Geometry check sheet. Reference: the model listing, model coordinates, mm. A direction names the side the tool comes from. Round coordinates to 2 decimals unless told otherwise and drop trailing zeros. Write each loop counter-clockwise with the first axis right and the second up, starting at its lowest first coordinate (ties: lowest second). Pieces come first, ordered by that corner, then holes. Notation, with made-up numbers: M 9.5,77 L 55.5,77 A27 cw 55.5,113 Z; hole C 79.5,6.25 d2. An arc over 180 degrees is marked long. Answer as CSV lines item,"result". Start each with the question number.
```python
from build123d import *

# Parameters (mm, degrees)
F1_DEPTH = 2
F3_DEPTH = 1


with BuildPart() as f1:
    # F0 (on Top) → F1 (new body)
    with BuildSketch(Plane.XY):
        Polygon((0, -11), (0, 0), (0, 11), (-2, 11), (-2, 2), (-8, 4.923089), (-8, 10.923089), (-12, 10.923089), (-12, 4.923089), (-29, 4.923089), (-46, 4.923089), (-46, 10.923089), (-50, 10.923089), (-50, 4.923089), (-60, 2), (-60, 10.923089), (-62, 10.923089), (-62, -10.923089), (-60, -10.923089), (-60, -2), (-50, -4.923089), (-50, -10.923089), (-46, -10.923089), (-46, -4.923089), (-29, -4.923089), (-12, -4.923089), (-12, -10.923089), (-8, -10.923089), (-8, -4.923089), (-2, -2), (-2, -11), align=None)
        Polygon((-60, 0), (-50, 2.923089), (-50, -2.923089), align=None, mode=Mode.SUBTRACT)
        Polygon((-12, 2.923089), (-12, 0), (-12, -2.923089), (-29, -2.923089), (-46, -2.923089), (-46, 0), (-46, 2.923089), (-29, 2.923089), align=None, mode=Mode.SUBTRACT)
        Polygon((-8, 2.923089), (-2, 0), (-8, -2.923089), (-8, 0), align=None, mode=Mode.SUBTRACT)
    extrude(amount=F1_DEPTH)

    # F2 (on face) → F3 (join)
    with BuildSketch(Plane.XY.offset(2)):
        with BuildLine():
            Line((-47.5, -3.076911), (-47.5, 2.923089))
            ThreePointArc((-47.5, 2.923089), (-48, 3.423089), (-48.5, 2.923089))
            Line((-48.5, 2.923089), (-48.5, -3.076911))
            ThreePointArc((-48.5, -3.076911), (-48, -3.576911), (-47.5, -3.076911))
        make_face()
        with BuildLine():
            Line((-9.5, -3.076911), (-9.5, 2.923089))
            ThreePointArc((-9.5, 2.923089), (-10, 3.423089), (-10.5, 2.923089))
            Line((-10.5, 2.923089), (-10.5, -3.076911))
            ThreePointArc((-10.5, -3.076911), (-10, -3.576911), (-9.5, -3.076911))
        make_face()
    extrude(amount=F3_DEPTH)


solid = f1.part
```
1) Section check B-B, the plane y = 6.5. Record the cut outline in (x, z), plus the area to 3 significant figures.
2) Section check C-C, the plane z = 0.65. Give the number of separate pieces and of enclosed holes in the cut face, plus the area to 3 significant figures.
3) Go/stop test with flat-tipped pins: pin 1 (1.6 mm diameter, centred on x = -60.5, z = 1.5, fed in from -Y); pin 2 (12 mm diameter, centred on x = -23, y = 1.5, fed in from +Z); pin 3 (0.6 mm diameter, centred on x = -21.5, z = 0.5, fed in from -Y). Record where each tip stops, or that it passes through.
4) Scan lines: line 1 (X direction, y = 9.5, z = 1); line 2 (Y direction, x = -31, z = 0.4); line 3 (X direction, y = 1.5, z = 2.7). Record each from-to range of solid material in increasing order. Write a range as from..to.
5) Mould release check, pull along X, two halves, no side actions. Record for faces 1 (the flat face through (-55.07, 1.44, 0.99)), 2 (the flat face through (-10, 0, 3)), 3 (the flat face through (-9.5, -0.1, 2.5)): released by +X, released by -X, zero draft, split by the parting line, or undercut.
6) Access from +Z, -Z, +X, -X, +Y, -Y to the whole of each face (thin tool, end or side, straight path). Record for faces 4 (the flat face through (-12, 8, 1)), 5 (the flat face through (-46, -8, 1)), 6 (the cylindrical face through (-9.989, 3.423, 2.493)), 7 (the cylindrical face through (-10.011, -3.577, 2.493)), 8 (the flat face through (-29, -2.923, 1)).
7) Section check A-A, the plane x = -37.5. Record the cut outline in (y, z), plus the area to 3 significant figures.
Results:
1,outline,"M -62,0 L -60,0 L -60,2 L -62,2 Z; M -50,0 L -46,0 L -46,2 L -50,2 Z; M -12,0 L -8,0 L -8,2 L -12,2 Z; M -2,0 L 0,0 L 0,2 L -2,2 Z"
1,area,"24.0 mm^2"
2,separate pieces,"1"
2,enclosed holes,"3"
2,area,"462 mm^2"
3,pin 1,"stops at y = -10.92"
3,pin 2,"stops at z = 2"
3,pin 3,"stops at y = -4.92"
4,line 1,"x = -62..-60, -50..-46, -12..-8, -2..0"
4,line 2,"y = -4.92..-2.92, 2.92..4.92"
4,line 3,"x = -48.5..-47.5, -10.5..-9.5"
5,face 1,"undercut"
5,face 2,"zero draft"
5,face 3,"released by +X"
6,face 4,"+Z, -Z, +Y"
6,face 5,"+Z, -Z, -Y"
6,face 6,"+Z, +Y"
6,face 7,"+Z, -Y"
6,face 8,"+Z, -Z"
7,outline,"M -4.92,0 L -2.92,0 L -2.92,2 L -4.92,2 Z; M 2.92,0 L 4.92,0 L 4.92,2 L 2.92,2 Z"
7,area,"8.00 mm^2"
